Here's how the part is built. I have some questions about the finished solid (model axes, mm). Face numbers are marked on the shaded views. A direction names the side the tool comes from. Coordinates: 2 decimals unless noted, no trailing zeros. Write each loop counter-clockwise with the first axis right and the second up, starting at its lowest first coordinate (ties: lowest second). Pieces come first, ordered by that corner, then holes.
Item 1: I want a section at C-C (y = 0). Please give me the cut outline in (x, z).
Item 2: I want a section at D-D (z = 68). Please give me the cut outline in (x, y), and give its area (3 significant figures).
Item 3: Please list where these lines run through material, in increasing order: line 1 (Z direction, x = 0, y = -8.35); line 2 (Z direction, x = 0, y = -7); line 3 (Z direction, x = 0, y = -9.1).
Item 4: I'm going to push flat-ended pins straight in: P1, Ø4, axis at y = -3.5, z = 9.5, coming from the -X side; P2, Ø2, axis at x = 0.5, y = 2.5, coming from the +Z side; P3, Ø3, axis at x = -0.5, z = 45.5, coming from the -Y side. Where does each tip first touch, or does it pass through?
Item 5: For the marked faces 4 and 5, which set-ups out of +Z, -Z, +X, -X, +Y, -Y let a thin tool reach every point of the face, with its end or its side?
Item 6: I want a section at B-B (x = 0). Please give me the cut outline in (y, z), and give its area (3 significant figures).
Item 7: I want a section at A-A (z = 60). Please give me the cut outline in (x, y).
Item 8: If we mould it in two halves opening along Y, with no side actions, what happens to the marked faces 1, 2 and 3? For each: pulls with the +Y half, pulls with the -Y half, needs draft (parallel to the pull), parting line crosses it, or undercut.
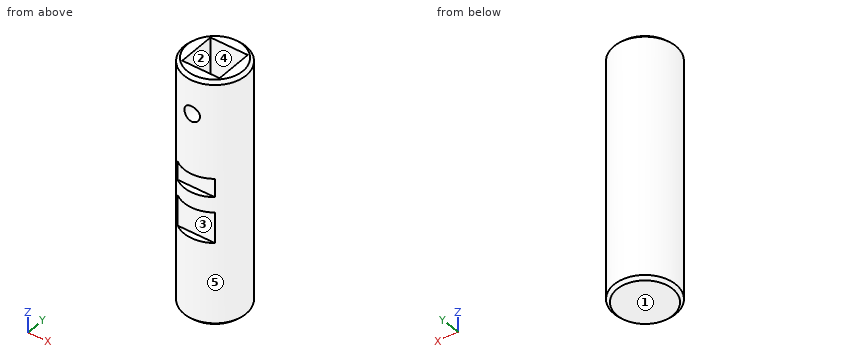
from build123d import *

# Parameters (mm, degrees)
F0_R     = 10
F1_DEPTH = 80
F2_W     = 12
F2_H     = 12
F3_DEPTH = 22
F6_D     = 5
F6_DEPTH = 12
F7_W     = 4
F7_H     = 6
F7_H_2   = 10
F8_DEPTH = 12.5
F9_SIZE  = 1


with BuildPart() as f1:
    # F0 (on Top) → F1 (new body)
    with BuildSketch(Plane.XY):
        Circle(F0_R)
    extrude(amount=F1_DEPTH)

    # F2 (on face) → F3 (cut)
    with BuildSketch(Plane.XY.offset(80)):
        Rectangle(F2_W, F2_H)
    extrude(amount=-F3_DEPTH, mode=Mode.SUBTRACT)

    # F6
    with Locations(Plane.XZ.offset(10)):
        with Locations((0, 68)):
            Hole(F6_D / 2, depth=F6_DEPTH)

    # F7 (on Right) → F8 (cut, symmetric)
    with BuildSketch(Plane.YZ):
        with Locations((-10, 45.3)):
            Rectangle(F7_W, F7_H)
        with Locations((-10, 32.3)):
            Rectangle(F7_W, F7_H_2)
    extrude(amount=F8_DEPTH, both=True, mode=Mode.SUBTRACT)

    # F9
    f9_edges = [f1.edges().sort_by_distance(p)[0] for p in [
        (-10, 0, 80),
        (-10, 0, 0),
    ]]
    chamfer(f9_edges, length=F9_SIZE)


solid = f1.part
Answer:
1. outline: (-10, 1) - (-9, 0) - (9, 0) - (10, 1) - (10, 79) - (9, 80) - (6, 80) - (6, 58) - (-6, 58) - (-6, 80) - (-9, 80) - (-10, 79) - close
2. outline: (-6, -6) - (-6, 6) - (6, 6) - (6, -6) - (2.5, -6) - (2.5, -9.68) arc R10 ccw (long way) to (-2.5, -9.68) - (-2.5, -6) - close
2. area: 151 mm2
3. line 1: z = 0 to 27.3, 37.3 to 42.3, 48.3 to 65.5, 70.5 to 80
3. line 2: z = 0 to 65.5, 70.5 to 80
3. line 3: z = 0.1 to 27.3, 37.3 to 42.3, 48.3 to 65.5, 70.5 to 79.9
4. P1: stops at x = -9.89
4. P2: stops at z = 58
4. P3: stops at y = -8
5. face 4: +Z
5. face 5: +Z, -Z
6. outline: (-10, 1) - (-9, 0) - (9, 0) - (10, 1) - (10, 79) - (9, 80) - (6, 80) - (6, 58) - (-6, 58) - (-6, 65.5) - (-10, 65.5) - (-10, 48.3) - (-8, 48.3) - (-8, 42.3) - (-10, 42.3) - (-10, 37.3) - (-8, 37.3) - (-8, 27.3) - (-10, 27.3) - close; (-10, 70.5) - (-6, 70.5) - (-6, 80) - (-9, 80) - (-10, 79) - close
6. area: 1,280 mm2
7. outline: circle Ø20 at (0, 0); hole (-6, -6) - (6, -6) - (6, 6) - (-6, 6) - close
8. face 1: needs draft
8. face 2: undercut
8. face 3: pulls with the -Y half
